Build history of the part. All positions in model axes, mm. Face numbers are marked on the shaded views. A direction names the side the tool comes from. Coordinates: 2 decimals unless noted, no trailing zeros. Write each loop counter-clockwise with the first axis right and the second up, starting at its lowest first coordinate (ties: lowest second). Pieces come first, ordered by that corner, then holes.
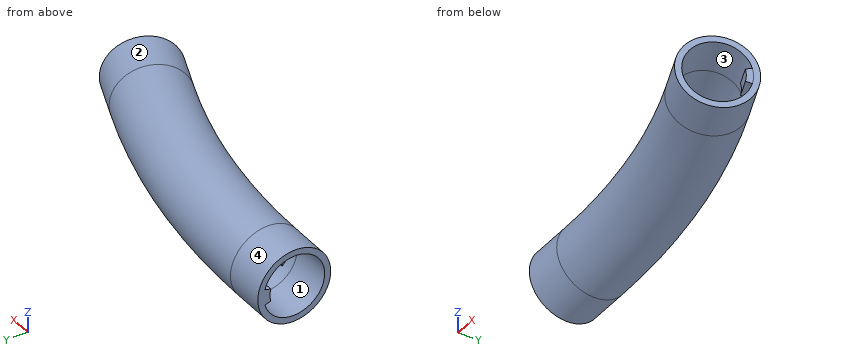
```python
from build123d import *

# Parameters (mm, degrees)
SKETCH3_R                                  = 9
SKETCH3_R_2                                = 7.5
BOSS_EXTRUDE3_START                        = -5
BOSS_EXTRUDE3_DEPTH                        = 5
BOSS_EXTRUDE4_DEPTH                        = 5
BOSS_EXTRUDE5_REACH                        = 138.641
BOSS_EXTRUDE5_END_MAJOR_RADIUS             = 154.759840898
BOSS_EXTRUDE5_END_MINOR_RADIUS             = 7.5
BOSS_EXTRUDE5_DIRECTION_2_REACH            = 138.641
BOSS_EXTRUDE5_DIRECTION_2_END_MAJOR_RADIUS = 154.759840898
BOSS_EXTRUDE5_DIRECTION_2_END_MINOR_RADIUS = 7.5


with BuildPart() as part:
    # Sweep1: sweep along a path in Sketch2path
    with BuildLine(Plane.XY) as sweep1_path:
        Line((78.462822432, 84.392774239), (69.224027107, 88.219608562))
        ThreePointArc((69.224027107, 88.219608562), (40.192147196, 97.026333052), (10, 100))
        Line((10, 100), (0, 100))
    # Sketch3 → Sweep1 (sweep)
    with BuildSketch(Plane(origin=(0, 0, 0), x_dir=(0, 0, -1), z_dir=(1, 0, 0))):
        with Locations((0, 100)):
            Circle(SKETCH3_R)
        with Locations((0, 100)):
            Circle(SKETCH3_R_2, mode=Mode.SUBTRACT)
    sweep(path=sweep1_path.line)

    # Sketch9 → Boss-Extrude3 (add)
    with BuildSketch(Plane(origin=(37.134856649, -15.381761261, 0), x_dir=(0, 0, -1), z_dir=(0.9238795325112893, -0.3826834323650841, 0)).offset(BOSS_EXTRUDE3_START)):
        with BuildLine():
            Line((-1.552914271, 113.79073397), (-1.941142838, 115.23962271))
            ThreePointArc((-1.941142838, 115.23962271), (0, 115.495179012), (1.941142838, 115.23962271))
            Line((1.941142838, 115.23962271), (1.552914271, 113.79073397))
            ThreePointArc((1.552914271, 113.79073397), (0, 113.995179012), (-1.552914271, 113.79073397))
        make_face()
    extrude(amount=BOSS_EXTRUDE3_DEPTH)

    # Sketch10 → Boss-Extrude4 (add)
    with BuildSketch(Plane.ZY):
        with BuildLine():
            Line((-1.552914271, 105.795554958), (-1.941142838, 107.244443697))
            ThreePointArc((-1.941142838, 107.244443697), (0, 107.5), (1.941142838, 107.244443697))
            Line((1.941142838, 107.244443697), (1.552914271, 105.795554958))
            ThreePointArc((1.552914271, 105.795554958), (0, 106), (-1.552914271, 105.795554958))
        make_face()
    extrude(amount=-BOSS_EXTRUDE4_DEPTH)

    # Boss-Extrude5: up to this torus (the profile starts inside it)
    boss_extrude5_end = Plane(origin=(10, -54.759840898, 0), z_dir=(0, 0, -1)) * Torus(BOSS_EXTRUDE5_END_MAJOR_RADIUS, BOSS_EXTRUDE5_END_MINOR_RADIUS, mode=Mode.PRIVATE)
    # Sketch12 → Boss-Extrude5 (add, up to the surface)
    with BuildSketch(Plane.XY, mode=Mode.PRIVATE) as boss_extrude5_sk1:
        with BuildLine():
            Line((12.604943408, 94.477267003), (12.570038595, 92.477571613))
            ThreePointArc((12.570038595, 92.477571613), (14.497096597, 92.431316661), (16.423384043, 92.359841262))
            Line((16.423384043, 92.359841262), (16.510622818, 94.357937705))
            ThreePointArc((16.510622818, 94.357937705), (14.558173623, 94.430383842), (12.604943408, 94.477267003))
        make_face()
    boss_extrude5_tool1 = extrude(boss_extrude5_sk1.sketch, amount=BOSS_EXTRUDE5_REACH, mode=Mode.PRIVATE) & boss_extrude5_end
    add(boss_extrude5_tool1.solids().sort_by_distance((14.527574, 93.428865, 0))[0])
    # Sketch12 → Boss-Extrude5 (add, up to the surface)
    with BuildSketch(Plane.XY, mode=Mode.PRIVATE) as boss_extrude5_sk2:
        with BuildLine():
            ThreePointArc((60.36583189, 83.619144932), (62.172841887, 82.948021298), (63.970912336, 82.253302132))
            Line((63.970912336, 82.253302132), (64.70391479, 84.114137268))
            ThreePointArc((64.70391479, 84.114137268), (62.881423963, 84.818291718), (61.049872177, 85.498530174))
            Line((61.049872177, 85.498530174), (60.36583189, 83.619144932))
        make_face()
    boss_extrude5_tool2 = extrude(boss_extrude5_sk2.sketch, amount=BOSS_EXTRUDE5_REACH, mode=Mode.PRIVATE) & boss_extrude5_end
    add(boss_extrude5_tool2.solids().sort_by_distance((62.526429, 83.8813, 0))[0])
    # Sketch12 → Boss-Extrude5 (add, up to the surface)
    with BuildSketch(Plane.XY, mode=Mode.PRIVATE) as boss_extrude5_sk3:
        with BuildLine():
            ThreePointArc((43.708421499, 103.960032742), (41.627954662, 104.38766443), (39.542068537, 104.788027012))
            Line((39.542068537, 104.788027012), (39.177935695, 102.821454544))
            ThreePointArc((39.177935695, 102.821454544), (41.238111377, 102.426026794), (43.29293457, 102.003666055))
            Line((43.29293457, 102.003666055), (43.708421499, 103.960032742))
        make_face()
    boss_extrude5_tool3 = extrude(boss_extrude5_sk3.sketch, amount=BOSS_EXTRUDE5_REACH, mode=Mode.PRIVATE) & boss_extrude5_end
    add(boss_extrude5_tool3.solids().sort_by_distance((41.432538, 103.404356, 0))[0])

    # Boss-Extrude5 direction 2: up to this torus (the profile starts inside it)
    boss_extrude5_direction_2_end = Plane(origin=(10, -54.759840898, 0), z_dir=(0, 0, -1)) * Torus(BOSS_EXTRUDE5_DIRECTION_2_END_MAJOR_RADIUS, BOSS_EXTRUDE5_DIRECTION_2_END_MINOR_RADIUS, mode=Mode.PRIVATE)
    # Sketch12 → Boss-Extrude5 direction 2 (add, up to the surface)
    with BuildSketch(Plane.XY, mode=Mode.PRIVATE) as boss_extrude5_direction_2_sk1:
        with BuildLine():
            Line((12.604943408, 94.477267003), (12.570038595, 92.477571613))
            ThreePointArc((12.570038595, 92.477571613), (14.497096597, 92.431316661), (16.423384043, 92.359841262))
            Line((16.423384043, 92.359841262), (16.510622818, 94.357937705))
            ThreePointArc((16.510622818, 94.357937705), (14.558173623, 94.430383842), (12.604943408, 94.477267003))
        make_face()
    boss_extrude5_direction_2_tool1 = extrude(boss_extrude5_direction_2_sk1.sketch, amount=-BOSS_EXTRUDE5_DIRECTION_2_REACH, mode=Mode.PRIVATE) & boss_extrude5_direction_2_end
    add(boss_extrude5_direction_2_tool1.solids().sort_by_distance((14.527574, 93.428865, 0))[0])
    # Sketch12 → Boss-Extrude5 direction 2 (add, up to the surface)
    with BuildSketch(Plane.XY, mode=Mode.PRIVATE) as boss_extrude5_direction_2_sk2:
        with BuildLine():
            ThreePointArc((60.36583189, 83.619144932), (62.172841887, 82.948021298), (63.970912336, 82.253302132))
            Line((63.970912336, 82.253302132), (64.70391479, 84.114137268))
            ThreePointArc((64.70391479, 84.114137268), (62.881423963, 84.818291718), (61.049872177, 85.498530174))
            Line((61.049872177, 85.498530174), (60.36583189, 83.619144932))
        make_face()
    boss_extrude5_direction_2_tool2 = extrude(boss_extrude5_direction_2_sk2.sketch, amount=-BOSS_EXTRUDE5_DIRECTION_2_REACH, mode=Mode.PRIVATE) & boss_extrude5_direction_2_end
    add(boss_extrude5_direction_2_tool2.solids().sort_by_distance((62.526429, 83.8813, 0))[0])
    # Sketch12 → Boss-Extrude5 direction 2 (add, up to the surface)
    with BuildSketch(Plane.XY, mode=Mode.PRIVATE) as boss_extrude5_direction_2_sk3:
        with BuildLine():
            ThreePointArc((43.708421499, 103.960032742), (41.627954662, 104.38766443), (39.542068537, 104.788027012))
            Line((39.542068537, 104.788027012), (39.177935695, 102.821454544))
            ThreePointArc((39.177935695, 102.821454544), (41.238111377, 102.426026794), (43.29293457, 102.003666055))
            Line((43.29293457, 102.003666055), (43.708421499, 103.960032742))
        make_face()
    boss_extrude5_direction_2_tool3 = extrude(boss_extrude5_direction_2_sk3.sketch, amount=-BOSS_EXTRUDE5_DIRECTION_2_REACH, mode=Mode.PRIVATE) & boss_extrude5_direction_2_end
    add(boss_extrude5_direction_2_tool3.solids().sort_by_distance((41.432538, 103.404356, 0))[0])


solid = part.part
```
1. Probe line 1 along Z through (x, y) = (7, 100); line 2 along Y through (x, z) = (3, 0); line 3 along Y through (x, z) = (71.5, 5.75). List the from-to ranges inside material, lowest first.
Computed values:
line 1: z = -9 to -7.5, 7.5 to 9
line 2: y = 91 to 92.5, 106 to 109
line 3: y = 79.78 to 82.06, 92.49 to 94.77
2. Saw through at A-A on z = 6.25. List the corners of the cut face in (x, y), plus the area to 3 significant figures.
Computed values:
outline: (0, 93.52) - (10, 93.52) arc R148.28 cw to (66.75, 82.24) - (75.98, 78.41) - (76.88, 80.56) - (67.64, 84.39) arc R150.61 ccw to (10, 95.85) - (0, 95.85) - close; (0, 104.15) - (10, 104.15) arc R158.91 cw to (70.81, 92.05) - (80.05, 88.22) - (80.94, 90.38) - (71.7, 94.2) arc R161.24 ccw to (10, 106.48) - (0, 106.48) - close
area: 376 mm2
3. 3-axis set-ups, long thin cutter, end or side, ignore diameter. For the marked faces 3 and 4: which of +Z, -Z, +X, -X, +Y, -Y reach the whole face in a straight line?
Computed values:
face 3: none
face 4: -X
4. Flat gauge pins, fed straight in: pin 1 (2 mm diameter, centred on x = 36.5, z = 0, fed in from +Y); pin 2 (1 mm diameter, centred on x = 70, y = 90, fed in from +Z); pin 3 (6 mm diameter, centred on x = 49, y = 85.5, fed in from +Z). Where does each tip first touch, or does it go through?
Computed values:
pin 1: stops at y = 107
pin 2: stops at z = 8.88
pin 3: stops at z = 6.54
5. Mould opens along Z. For the marked faces 1 and 2 say: +Z half, -Z half, draft (parallel to the pull), parting line (faces both ways), or undercut.
Computed values:
face 1: undercut
face 2: parting line
